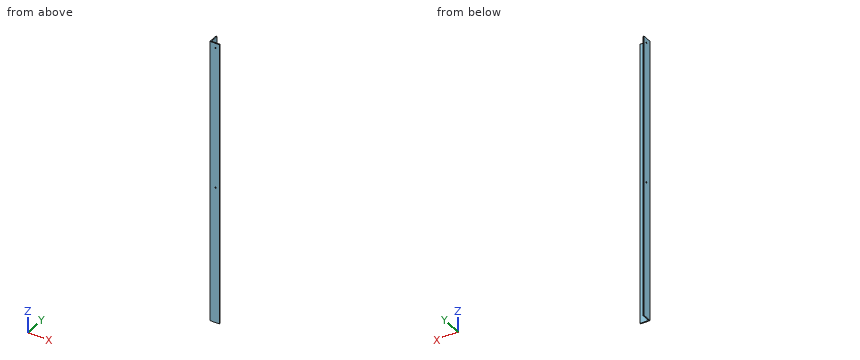
Autodesk Inventor part; units mm, degrees
ref_plane "YZ Plane" through (0, 0, 0) normal (1, 0, 0) x (0, 1, 0)
ref_plane "XZ Plane" through (0, 0, 0) normal (0, 1, 0) x (-1, 0, 0)
ref_plane "XY Plane" through (0, 0, 0) normal (0, 0, 1) x (1, 0, 0)
sketch "Sketch1" plane through (0, 0, 0) normal (0, 0, 1) x (1, 0, 0)
  line L0 (0, 0) -> (30, 0)
  line L1 (30, 0) -> (30, 3)
  line L2 (30, 3) -> (3, 3)
  line L3 (3, 3) -> (3, 30)
  line L4 (3, 30) -> (0, 30)
  line L5 (0, 30) -> (0, 0)
  dimension "d0" = 3
  dimension "d1" = 3
  dimension "d2" = 30
  dimension "d3" = 30
extrude "Extrusion1" add sketch "Sketch1" along normal blind 900
sketch "Sketch2" plane through (3, 3, 900) normal (0, 1, 0) x (1, 0, 0)
  line L0 (0, 900) -> (0, 0)
  line L1 (27, 0) -> (0, 0)
  point P0 (-3, 900)
  point P1 (15, 15)
  point P2 (15, 465)
  point P3 (15, 915)
  point P4 (15, 1365)
  dimension "d6" = 15
  dimension "d7" = 15
  dimension "d8" = 27
  dimension "d9" = 15
  dimension "d10" = 450
  dimension "d11" = 450
  dimension "d12" = 15
  dimension "d13" = 450
  dimension "d14" = 15
hole "Hole1" at (18, 3, 885) at (18, 3, 435) at (18, 3, -15) at (18, 3, -465) direction (0, -1, 0) diameter 3.81 end through all
sketch "Sketch3" plane through (3, 30, 900) normal (1, 0, 0) x (0, 0, -1)
  line L0 (0, -27) -> (0, 0)
  line L1 (900, -27) -> (0, -27)
  point P0 (900, -30)
  point P1 (15, -12)
  point P2 (465, -12)
  point P3 (915, -12)
  point P4 (1365, -12)
  dimension "d22" = 15
  dimension "d23" = 15
  dimension "d24" = 15
  dimension "d25" = 450
  dimension "d26" = 450
  dimension "d27" = 15
  dimension "d28" = 450
  dimension "d29" = 15
hole "Hole2" at (3, 18, 885) at (3, 18, 435) at (3, 18, -15) at (3, 18, -465) direction (-1, 0, 0) diameter 3.81 end through all
equation "\"d0\" = Thickness"
equation "\"d1\" = Thickness"
equation "\"d2\" = Width"
equation "\"d3\" = Width"
equation "\"d4\" = Height"
equation "\"Width\" = 30"
equation "\"Thickness\" = 3"
equation "\"Height\" = 900"
equation "\"HoleDistance\" = 15"
properties part number "corner90"
Geometry: final body of the model. Coordinates: model frame, mm. Coordinates: 2 decimals unless noted, no trailing zeros. Order: outer loops, then holes, each group sorted by start corner. A loop starts at its lowest first (then second) coordinate and runs counter-clockwise, first axis right, second up. Notation, with made-up numbers: (-5.5, 84.25) -> (27.5, 84.25) arc R5 cw to (27.5, 89.25) -> close; hole circle Ø9 at (-37.5, -27.5). An arc over 180 degrees is marked (long way). Use CSV: the item, a comma, the result in double quotes.
1) Pin query (flat end, axial travel): pin 1 Ø5 at (y, z) = (17.5, 213) entering from +X; pin 2 Ø5 at (x, z) = (18, 885) entering from +Y; pin 3 Ø12 at (x, y) = (10, 19) entering from -Z. Return the tip coordinate at first contact, or that it passes through.
Findings:
pin 1,"stops at x = 3"
pin 2,"stops at y = 3"
pin 3,"passes through"
2) Line query: line 1 (Z direction, x = 18, y = 1.15) (3 decimals); line 2 (Y direction, x = 0.9, z = 435) (3 decimals). Output: solid intervals per line, ascending.
Findings:
line 1,"z = 0 to 433.095, 436.905 to 883.095, 886.905 to 900"
line 2,"y = 0 to 16.095, 19.905 to 30"
3) Section A-A on z = 755.5. Output: boundary loops of the cut face in (x, y), then the cut area to 3 significant figures.
Findings:
outline,"(0, 0) -> (30, 0) -> (30, 3) -> (3, 3) -> (3, 30) -> (0, 30) -> close"
area,"171 mm^2"
